Read the model definition and answer for the solid it produces. Units are mm, in the model's axes. Coordinates: 2 decimals unless noted, no trailing zeros.
Item 1: Each of these flat-tipped pins is pushed along its axis until it touches: P1, Ø1, axis at y = 16, z = 4, coming from the -X side; P2, Ø1, axis at y = 14.5, z = 1.5, coming from the -X side; P3, Ø2.5, axis at y = 0.5, z = 3.5, coming from the -X side. Where does it stop, or does it pass through?
Item 2: Section A-A (z = 2.4) is taken. State how many separate pieces and enclosed holes the cut face has, then the cut area to 3 significant figures.
Item 3: Straight lines are drawn through the part: probe 1 along Y at (x, z) = (5, 3.9); probe 2 along Y at (x, z) = (-9, 4.7); probe 3 along Y at (x, z) = (-54.5, 0.4). For each, find the intervals that lie inside material, in ascending order.
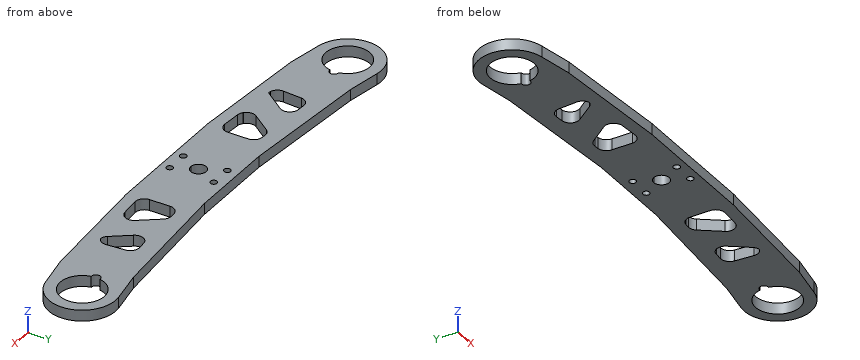
from build123d import *

# Parameters (mm, degrees)
IZIM1_R                     = 1.5
Y_KSEKLIK_EKSTR_ZYON3_DEPTH = 5
KES_EKSTR_ZYON3_DEPTH       = 16
RADYUS1_R                   = 4
RADYUS1_OF_AYNALAMA1_R      = 4


with BuildPart() as part:
    # Çizim1 → Yükseklik-Ekstrüzyon3 (new body)
    with BuildSketch(Plane.XY):
        with BuildLine():
            Line((0, 15.000289945), (20, 15.000289945))
            Line((20, 15.000289945), (79.814271892, 19.717585574))
            Line((79.814271892, 19.717585574), (95.039910294, 22.402276423))
            ThreePointArc((95.039910294, 22.402276423), (112.619627342, 9.95914701), (99.998384592, -7.493135147))
            Line((99.998384592, -7.493135147), (84.9128284, -10.282704371))
            Line((84.9128284, -10.282704371), (30.084066985, -14.204712795))
            Line((30.084066985, -14.204712795), (0, -14.204712795))
            Line((0, -14.204712795), (0, -3.5))
            ThreePointArc((0, -3.5), (3.5, 0), (0, 3.5))
            Line((0, 3.5), (0, 15.000289945))
        make_face()
        with Locations((5, 10.000289945)):
            Circle(IZIM1_R, mode=Mode.SUBTRACT)
        with Locations((5, -10)):
            Circle(IZIM1_R, mode=Mode.SUBTRACT)
    y_kseklik_ekstr_zyon3 = extrude(amount=Y_KSEKLIK_EKSTR_ZYON3_DEPTH)

    # Çizim2 → Kes-Ekstrüzyon3 (cut)
    with BuildSketch(Plane.XY):
        with BuildLine():
            ThreePointArc((87.871148736, 5.489806807), (107.671148736, 7.479781681), (87.871148736, 9.469756555))
            ThreePointArc((87.871148736, 9.469756555), (85.671148736, 7.479781681), (87.871148736, 5.489806807))
        make_face()
        Polygon((65.565337221, -5.727765324), (64.37597588, 10.765231948), (49.583112015, 9.598582086), (61.257040732, -6.035946189), align=None)
        Polygon((42.731699056, -7.748306299), (46.735341753, -4.32569838), (36.65049886, 9.180616861), (28.695940883, 8.553274918), (28.695940883, -8.752311503), align=None)
    kes_ekstr_zyon3 = extrude(amount=KES_EKSTR_ZYON3_DEPTH, mode=Mode.SUBTRACT)

    # Radyus1
    # the kernel refuses this fillet: 4 mm, written as the material it adds along each edge
    with BuildSketch(Plane(origin=(28.695940883, -8.752311503, 0), x_dir=(0.9974513663147316, 0.07134964496670468, 0), z_dir=(0, 0, 1))) as radyus1_piece_1:
        with BuildLine():
            CenterArc((RADYUS1_R * 1.07408709953, RADYUS1_R), RADYUS1_R, 175.908489963, 94.091510037)
            Line((RADYUS1_R * 0.0766357332147, RADYUS1_R * 1.07134964497), (0, 0))
            Line((0, 0), (RADYUS1_R * 1.07408709953, 0))
        make_face()
    extrude(amount=5)
    with BuildSketch(Plane(origin=(64.37597588, 10.765231948, 0), x_dir=(-0.9969045315308735, -0.0786215938099059, 0), z_dir=(0, 0, 1))) as radyus1_piece_2:
        with BuildLine():
            CenterArc((RADYUS1_R * 1.0067369642, RADYUS1_R), RADYUS1_R, 179.615297698, 90.384702302)
            Line((RADYUS1_R * 0.00675950517271, RADYUS1_R * 1.00671427137), (0, 0))
            Line((0, 0), (RADYUS1_R * 1.0067369642, 0))
        make_face()
    extrude(amount=5)
    with BuildSketch(Plane(origin=(49.583112015, 9.598582086, 0), x_dir=(0.5982940894650635, -0.8012765955094225, 0), z_dir=(0, 0, 1))) as radyus1_piece_3:
        with BuildLine():
            CenterArc((RADYUS1_R * 1.81293545135, RADYUS1_R), RADYUS1_R, 147.761521051, 122.238478949)
            Line((RADYUS1_R * 0.967100347397, RADYUS1_R * 1.53344444595), (0, 0))
            Line((0, 0), (RADYUS1_R * 1.81293545135, 0))
        make_face()
    extrude(amount=5)
    with BuildSketch(Plane(origin=(65.565337221, -5.727765324, 0), x_dir=(-0.9974513663147317, -0.07134964496670451, 0), z_dir=(0, 0, 1))) as radyus1_piece_4:
        with BuildLine():
            CenterArc((RADYUS1_R * 1.0005783418, -RADYUS1_R), RADYUS1_R, 90, 90.033126964)
            Line((RADYUS1_R * 0.000578508947597, -RADYUS1_R * 1.00057817457), (0, 0))
            Line((0, 0), (RADYUS1_R * 1.0005783418, 0))
        make_face()
    extrude(amount=5)
    with BuildSketch(Plane(origin=(46.735341753, -4.32569838, 0), x_dir=(-0.5982940894650634, 0.8012765955094225, 0), z_dir=(0, 0, 1))) as radyus1_piece_5:
        with BuildLine():
            CenterArc((RADYUS1_R * 0.936136482984, RADYUS1_R), RADYUS1_R, 183.778435906, 86.221564094)
            Line((-RADYUS1_R * 0.0616898577771, RADYUS1_R * 0.934101641269), (0, 0))
            Line((0, 0), (RADYUS1_R * 0.936136482984, 0))
        make_face()
    extrude(amount=5)
    with BuildSketch(Plane(origin=(36.65049886, 9.180616861, 0), x_dir=(-0.9969045315308735, -0.07862159380990552, 0), z_dir=(0, 0, 1))) as radyus1_piece_6:
        with BuildLine():
            CenterArc((RADYUS1_R * 0.551591618585, RADYUS1_R), RADYUS1_R, 212.238478949, 57.761521051)
            Line((-RADYUS1_R * 0.294243485369, RADYUS1_R * 0.466555554046), (0, 0))
            Line((0, 0), (RADYUS1_R * 0.551591618585, 0))
        make_face()
    extrude(amount=5)
    with BuildSketch(Plane(origin=(28.695940883, 8.553274918, 0), x_dir=(0, -1, 0), z_dir=(0, 0, 1))) as radyus1_piece_7:
        with BuildLine():
            CenterArc((RADYUS1_R * 0.924239359987, RADYUS1_R), RADYUS1_R, 184.509339304, 85.490660696)
            Line((-RADYUS1_R * 0.072665171544, RADYUS1_R * 0.92137840619), (0, 0))
            Line((0, 0), (RADYUS1_R * 0.924239359987, 0))
        make_face()
    extrude(amount=5)
    with BuildSketch(Plane(origin=(42.731699056, -7.748306299, 0), x_dir=(-0.9974513663147319, -0.07134964496670451, 0), z_dir=(0, 0, 1))) as radyus1_piece_8:
        with BuildLine():
            CenterArc((RADYUS1_R * 0.32911927964, -RADYUS1_R), RADYUS1_R, 90, 36.434744123)
            Line((-RADYUS1_R * 0.26478758489, -RADYUS1_R * 0.195466199427), (0, 0))
            Line((0, 0), (RADYUS1_R * 0.32911927964, 0))
        make_face()
    extrude(amount=5)
    with BuildSketch(Plane(origin=(61.257040732, -6.035946189, 0), x_dir=(0.9974513663147319, 0.07134964496670383, 0), z_dir=(0, 0, 1))) as radyus1_piece_9:
        with BuildLine():
            CenterArc((RADYUS1_R * 0.546845511805, RADYUS1_R), RADYUS1_R, 212.656308216, 57.343691784)
            Line((-RADYUS1_R * 0.295076994051, RADYUS1_R * 0.460401543615), (0, 0))
            Line((0, 0), (RADYUS1_R * 0.546845511805, 0))
        make_face()
    extrude(amount=5)

    # Aynalama1: Yükseklik-Ekstrüzyon3, Kes-Ekstrüzyon3 across plane
    add(y_kseklik_ekstr_zyon3.mirror(Plane(origin=(0, 0, 0), x_dir=(0, 0, 1), z_dir=(1, 0, 0))))
    add(kes_ekstr_zyon3.mirror(Plane(origin=(0, 0, 0), x_dir=(0, 0, 1), z_dir=(1, 0, 0))), mode=Mode.SUBTRACT)

    # Radyus1 of Aynalama1
    # the kernel refuses this fillet: 4 mm, written as the material it adds along each edge
    with BuildSketch(Plane(origin=(-28.695940883, -8.752311503, 0), x_dir=(0, 1, 0), z_dir=(0, 0, 1))) as radyus1_of_aynalama1_piece_1:
        with BuildLine():
            CenterArc((RADYUS1_OF_AYNALAMA1_R * 1.07408709953, RADYUS1_OF_AYNALAMA1_R), RADYUS1_OF_AYNALAMA1_R, 175.908489963, 94.091510037)
            Line((RADYUS1_OF_AYNALAMA1_R * 0.0766357332147, RADYUS1_OF_AYNALAMA1_R * 1.07134964497), (0, 0))
            Line((0, 0), (RADYUS1_OF_AYNALAMA1_R * 1.07408709953, 0))
        make_face()
    extrude(amount=5)
    with BuildSketch(Plane(origin=(-64.37597588, 10.765231948, 0), x_dir=(-0.0719263340510189, -0.9974099470478431, 0), z_dir=(0, 0, 1))) as radyus1_of_aynalama1_piece_2:
        with BuildLine():
            CenterArc((RADYUS1_OF_AYNALAMA1_R * 1.0067369642, RADYUS1_OF_AYNALAMA1_R), RADYUS1_OF_AYNALAMA1_R, 179.615297698, 90.384702302)
            Line((RADYUS1_OF_AYNALAMA1_R * 0.00675950517271, RADYUS1_OF_AYNALAMA1_R * 1.00671427137), (0, 0))
            Line((0, 0), (RADYUS1_OF_AYNALAMA1_R * 1.0067369642, 0))
        make_face()
    extrude(amount=5)
    with BuildSketch(Plane(origin=(-49.583112015, 9.598582086, 0), x_dir=(-0.9969045315308733, 0.07862159380990602, 0), z_dir=(0, 0, 1))) as radyus1_of_aynalama1_piece_3:
        with BuildLine():
            CenterArc((RADYUS1_OF_AYNALAMA1_R * 1.81293545135, RADYUS1_OF_AYNALAMA1_R), RADYUS1_OF_AYNALAMA1_R, 147.761521051, 122.238478949)
            Line((RADYUS1_OF_AYNALAMA1_R * 0.967100347397, RADYUS1_OF_AYNALAMA1_R * 1.53344444595), (0, 0))
            Line((0, 0), (RADYUS1_OF_AYNALAMA1_R * 1.81293545135, 0))
        make_face()
    extrude(amount=5)
    with BuildSketch(Plane(origin=(-65.565337221, -5.727765324, 0), x_dir=(0.07192633405101899, 0.9974099470478431, 0), z_dir=(0, 0, 1))) as radyus1_of_aynalama1_piece_4:
        with BuildLine():
            CenterArc((RADYUS1_OF_AYNALAMA1_R * 1.0005783418, -RADYUS1_OF_AYNALAMA1_R), RADYUS1_OF_AYNALAMA1_R, 90, 90.033126964)
            Line((RADYUS1_OF_AYNALAMA1_R * 0.000578508947597, -RADYUS1_OF_AYNALAMA1_R * 1.00057817457), (0, 0))
            Line((0, 0), (RADYUS1_OF_AYNALAMA1_R * 1.0005783418, 0))
        make_face()
    extrude(amount=5)
    with BuildSketch(Plane(origin=(-46.735341753, -4.32569838, 0), x_dir=(0.7601082947002413, -0.6497964145237269, 0), z_dir=(0, 0, 1))) as radyus1_of_aynalama1_piece_5:
        with BuildLine():
            CenterArc((RADYUS1_OF_AYNALAMA1_R * 0.936136482984, RADYUS1_OF_AYNALAMA1_R), RADYUS1_OF_AYNALAMA1_R, 183.778435906, 86.221564094)
            Line((-RADYUS1_OF_AYNALAMA1_R * 0.0616898577771, RADYUS1_OF_AYNALAMA1_R * 0.934101641269), (0, 0))
            Line((0, 0), (RADYUS1_OF_AYNALAMA1_R * 0.936136482984, 0))
        make_face()
    extrude(amount=5)
    with BuildSketch(Plane(origin=(-36.65049886, 9.180616861, 0), x_dir=(-0.5982940894650631, -0.8012765955094229, 0), z_dir=(0, 0, 1))) as radyus1_of_aynalama1_piece_6:
        with BuildLine():
            CenterArc((RADYUS1_OF_AYNALAMA1_R * 0.551591618585, RADYUS1_OF_AYNALAMA1_R), RADYUS1_OF_AYNALAMA1_R, 212.238478949, 57.761521051)
            Line((-RADYUS1_OF_AYNALAMA1_R * 0.294243485369, RADYUS1_OF_AYNALAMA1_R * 0.466555554046), (0, 0))
            Line((0, 0), (RADYUS1_OF_AYNALAMA1_R * 0.551591618585, 0))
        make_face()
    extrude(amount=5)
    with BuildSketch(Plane(origin=(-28.695940883, 8.553274918, 0), x_dir=(-0.9969045315308733, 0.07862159380990584, 0), z_dir=(0, 0, 1))) as radyus1_of_aynalama1_piece_7:
        with BuildLine():
            CenterArc((RADYUS1_OF_AYNALAMA1_R * 0.924239359987, RADYUS1_OF_AYNALAMA1_R), RADYUS1_OF_AYNALAMA1_R, 184.509339304, 85.490660696)
            Line((-RADYUS1_OF_AYNALAMA1_R * 0.072665171544, RADYUS1_OF_AYNALAMA1_R * 0.92137840619), (0, 0))
            Line((0, 0), (RADYUS1_OF_AYNALAMA1_R * 0.924239359987, 0))
        make_face()
    extrude(amount=5)
    with BuildSketch(Plane(origin=(-42.731699056, -7.748306299, 0), x_dir=(-0.7601082947002398, 0.6497964145237288, 0), z_dir=(0, 0, 1))) as radyus1_of_aynalama1_piece_8:
        with BuildLine():
            CenterArc((RADYUS1_OF_AYNALAMA1_R * 0.32911927964, -RADYUS1_OF_AYNALAMA1_R), RADYUS1_OF_AYNALAMA1_R, 90, 36.434744123)
            Line((-RADYUS1_OF_AYNALAMA1_R * 0.26478758489, -RADYUS1_OF_AYNALAMA1_R * 0.195466199427), (0, 0))
            Line((0, 0), (RADYUS1_OF_AYNALAMA1_R * 0.32911927964, 0))
        make_face()
    extrude(amount=5)
    with BuildSketch(Plane(origin=(-61.257040732, -6.035946189, 0), x_dir=(0.5982940894650624, 0.8012765955094232, 0), z_dir=(0, 0, 1))) as radyus1_of_aynalama1_piece_9:
        with BuildLine():
            CenterArc((RADYUS1_OF_AYNALAMA1_R * 0.546845511805, RADYUS1_OF_AYNALAMA1_R), RADYUS1_OF_AYNALAMA1_R, 212.656308216, 57.343691784)
            Line((-RADYUS1_OF_AYNALAMA1_R * 0.295076994051, RADYUS1_OF_AYNALAMA1_R * 0.460401543615), (0, 0))
            Line((0, 0), (RADYUS1_OF_AYNALAMA1_R * 0.546845511805, 0))
        make_face()
    extrude(amount=5)


solid = part.part
Established:
1. P1: stops at x = -110.53
1. P2: stops at x = -111.35
1. P3: stops at x = -111.7
2. separate pieces: 1
2. enclosed holes: 11
2. area: 5,150 mm2
3. probe 1: y = -14.2 to -11.5, -8.5 to 8.5, 11.5 to 15
3. probe 2: y = -14.2 to 15
3. probe 3: y = -12.46 to 3.01, 9.2 to 17.72
